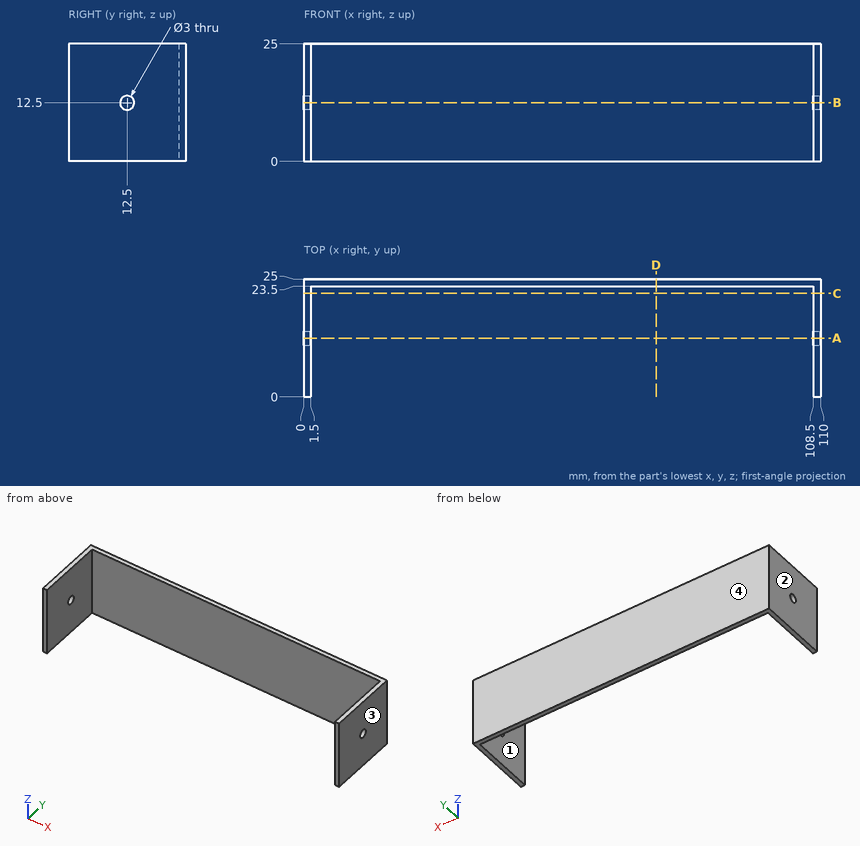
Check sheet for the drawn part. Datum: minimum x, y, z corner. Units: mm. Coordinates: 2 decimals unless noted, no trailing zeros. Order: outer loops, then holes, each group sorted by start corner. A loop starts at its lowest first (then second) coordinate and runs counter-clockwise, first axis right, second up. Notation, with made-up numbers: M 80.5,-38.5 L 121.5,-38.5 A10 cw 121.5,-20.5 Z; hole C 63,-10 d9. An arc over 180 degrees is marked long. One line per question, with ' | ' between items. Start each with the question number.
Item 1: Sectioned sample at B-B on z = 12.5. Record the cut outline in (x, y).
Item 2: Sectioned sample at D-D on x = 75. Record the cut outline in (y, z).
Item 3: Gauge pin test, flat end, axial feed: P1, Ø10, axis at x = 56, z = 12, coming from the -Y side. Record the tip position at first contact, or that the pin passes through.
Item 4: Mould release check, pull along X, two halves, no side actions. Record for the marked faces 1, 2, 3 and 4: pulls with the +X half, pulls with the -X half, needs draft (parallel to the pull), parting line crosses it, or undercut.
Item 5: Sectioned sample at C-C on y = 22. Record the cut outline in (x, z).
Item 6: Material ranges on line 1 (Y direction, x = 0.8, z = 12.5); line 2 (X direction, y = 17.25, z = 10); line 3 (Y direction, x = 81, z = 13.5), recorded low to high.
Item 7: Sectioned sample at A-A on y = 12.5. Record the cut outline in (x, z).
Answer below:
1) outline: M 0,0 L 1.5,0 L 1.5,11 L 0,11 Z; M 0,14 L 1.5,14 L 1.5,23.5 L 108.5,23.5 L 108.5,14 L 110,14 L 110,25 L 0,25 Z; M 108.5,0 L 110,0 L 110,11 L 108.5,11 Z
2) outline: M 23.5,0 L 25,0 L 25,25 L 23.5,25 Z
3) P1: stops at y = 23.5
4) face 1: undercut | face 2: pulls with the -X half | face 3: pulls with the +X half | face 4: needs draft
5) outline: M 0,0 L 1.5,0 L 1.5,25 L 0,25 Z; M 108.5,0 L 110,0 L 110,25 L 108.5,25 Z
6) line 1: y = 0 to 11, 14 to 25 | line 2: x = 0 to 1.5, 108.5 to 110 | line 3: y = 23.5 to 25
7) outline: M 0,0 L 1.5,0 L 1.5,11 L 0,11 Z; M 0,14 L 1.5,14 L 1.5,25 L 0,25 Z; M 108.5,0 L 110,0 L 110,11 L 108.5,11 Z; M 108.5,14 L 110,14 L 110,25 L 108.5,25 Z
